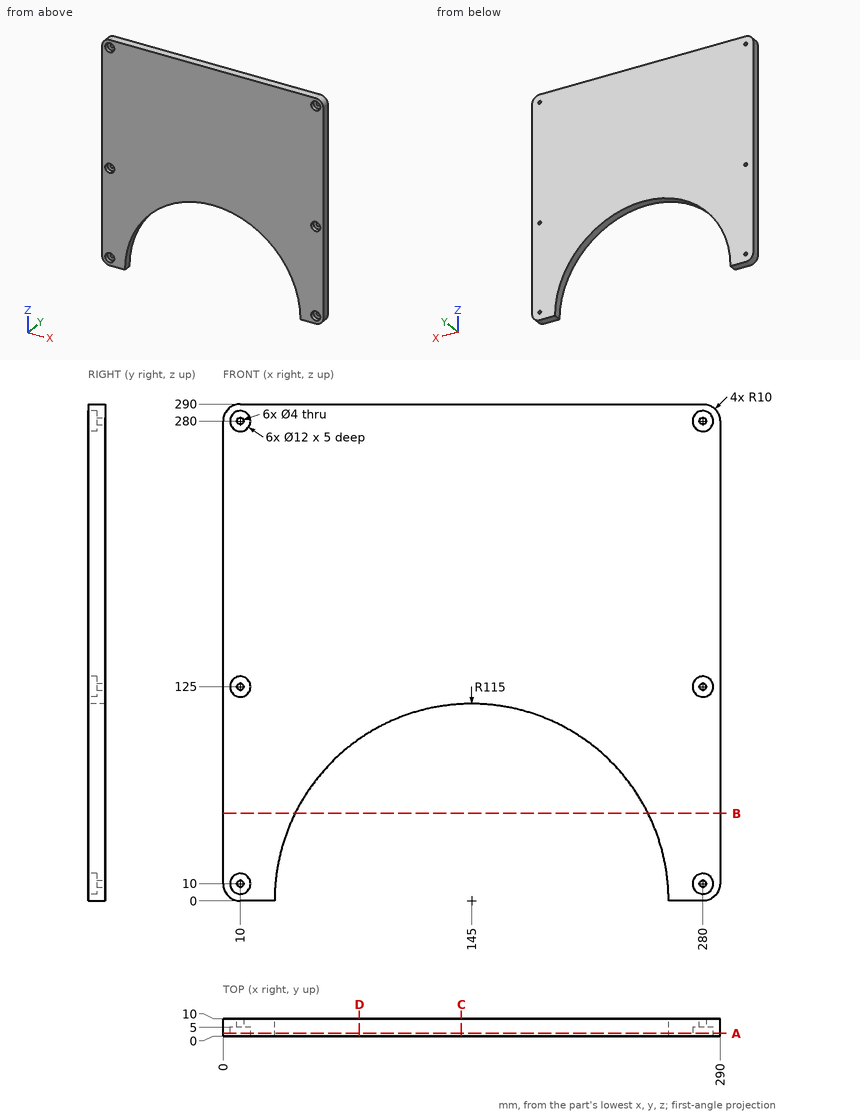
Answer from the drawing. Dimensions are ordinates in mm from the lowest x, y and z of the part. Give positions to 0.01 mm unless a question says otherwise; leave off trailing zeros. Loops run counter-clockwise (first coordinate to the right, second up) from the corner with the lowest first, then second, coordinate; pieces in that order, holes last. Notation, with made-up numbers: (-35, 81) -> (22, 81) arc R22 ccw to (22, 116) -> close; hole circle Ø6 at (-7, 72). An arc over 180 degrees is marked (long way). Answer as CSV lines item,"result".
Item 1: Consider line 1 (Z direction, x = 10, y = 7.4); line 2 (X direction, y = 8.65, z = 125); line 3 (X direction, y = 1.65, z = 125). Determine where each line is inside the solid, lowest interval first. Write a range as [from, to].
Returned:
line 1,"z = [0, 8], [12, 123], [127, 278], [282, 290]"
line 2,"x = [0, 8], [12, 278], [282, 290]"
line 3,"x = [0, 4], [16, 274], [286, 290]"
Item 2: Find section D-D on x = 79.5. Give the vertices of the cut face in (y, z), plus the area to 3 significant figures.
Returned:
outline,"(0, 94.52) -> (10, 94.52) -> (10, 290) -> (0, 290) -> close"
area,"1,950 mm²"
Item 3: This flat-tipped pin is pushed along its axis until it touches: pin 1 (6 mm diameter, centred on x = 281.5, z = 122.5, fed in from -Y). Where does it stop, or does it pass through?
Returned:
pin 1,"stops at y = 5"
Item 4: Find section A-A on y = 1.5. Give the vertices of the cut face in (x, z).
Returned:
outline,"(0, 10) arc R10 ccw to (10, 0) -> (30, 0) arc R115 cw to (260, 0) -> (280, 0) arc R10 ccw to (290, 10) -> (290, 280) arc R10 ccw to (280, 290) -> (10, 290) arc R10 ccw to (0, 280) -> close; hole circle Ø12 at (10, 10); hole circle Ø12 at (10, 125); hole circle Ø12 at (10, 280); hole circle Ø12 at (280, 10); hole circle Ø12 at (280, 125); hole circle Ø12 at (280, 280)"
Item 5: Find section C-C on x = 139. Give the vertices of the cut face in (y, z).
Returned:
outline,"(0, 114.84) -> (10, 114.84) -> (10, 290) -> (0, 290) -> close"
Item 6: Find section B-B on z = 51. Give the vertices of the cut face in (x, y).
Returned:
outline,"(0, 0) -> (41.93, 0) -> (41.93, 10) -> (0, 10) -> close; (248.07, 0) -> (290, 0) -> (290, 10) -> (248.07, 10) -> close"
